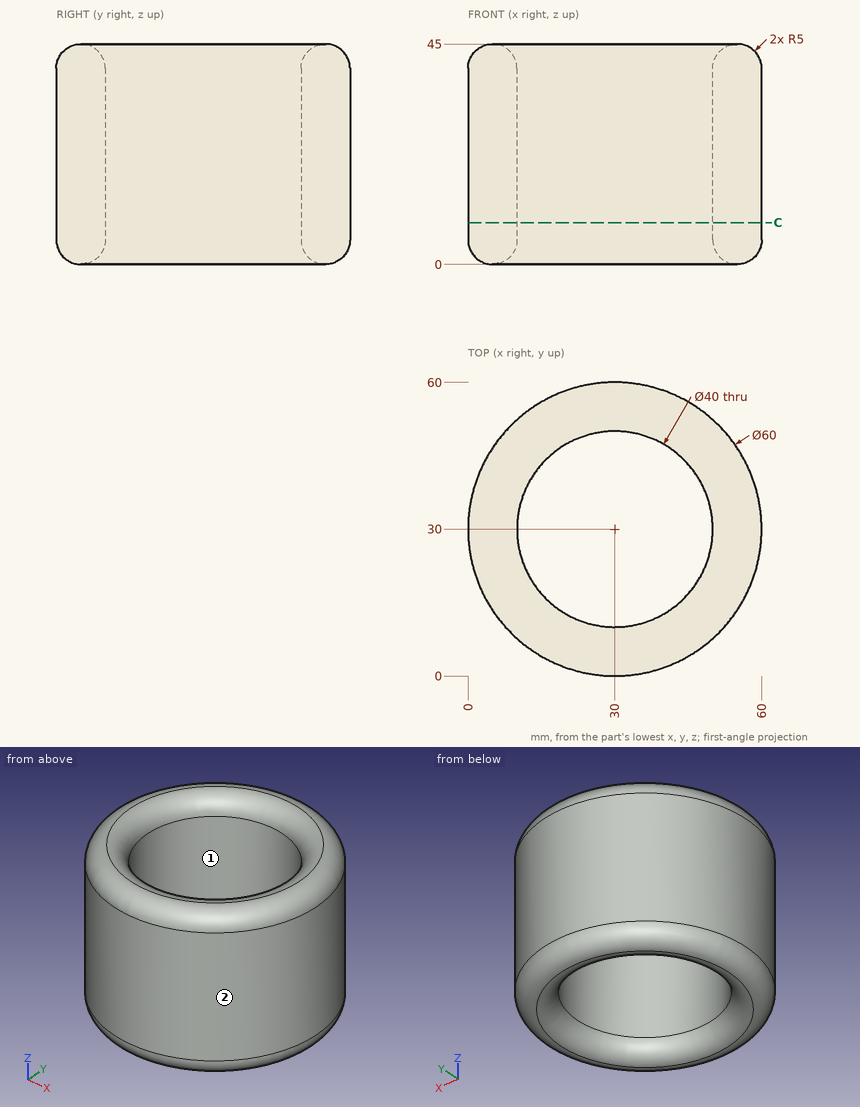
Source: three-view drawing plus pictorial views. Frame: mm from the lowest corner of the part. Give positions to 0.01 mm unless a question says otherwise; leave off trailing zeros. Write each loop counter-clockwise with the first axis right and the second up, starting at its lowest first coordinate (ties: lowest second). Pieces come first, ordered by that corner, then holes.
(1) Mould query, pull axis Y, two halves, no side actions, for the marked faces 1 and 2. Classes: released by +Y, released by -Y, zero draft, split by the parting line, or undercut.
(2) Ray query, line 1 (X direction, y = 29.5, z = 26); line 2 (Y direction, x = 30, z = 21); line 3 (X direction, y = 41.5, z = 15). Return the intervals inside material, ascending.
(3) First-contact query: P1, Ø1.5, axis at x = 52, y = 30.5, coming from the +Z side; P2, Ø4, axis at x = 21, z = 26, coming from the +Y side; P3, Ø2, axis at y = 33.5, z = 38, coming from the +X side; P4, Ø24, axis at x = 30, y = 30, coming from the -Z side. Flat tips, straight axial feed; report the tip coordinate or a pass-through.
(4) Cut plane C-C, the plane z = 8.5. Return loops of the section in (x, y).
Values follow:
1. face 1: undercut
1. face 2: split by the parting line
2. line 1: x = 0 to 10.01, 49.99 to 60
2. line 2: y = 0 to 10, 50 to 60
2. line 3: x = 2.29 to 13.64, 46.36 to 57.71
3. P1: stops at z = 44.47
3. P2: stops at y = 59.17
3. P3: stops at x = 59.9
3. P4: passes through
4. outline: circle Ø60 at (30, 30); hole circle Ø40 at (30, 30)
